```python
from build123d import *

# Parameters (mm, degrees)
SKETCH1_R           = 3
BOSS_EXTRUDE1_DEPTH = 10
BOSS_EXTRUDE2_START = -300
SKETCH2_R           = 3
BOSS_EXTRUDE2_DEPTH = 5
BOSS_EXTRUDE3_START = -270
SKETCH2_2_R         = 3
BOSS_EXTRUDE3_DEPTH = 5
SKETCH3_W           = 18
SKETCH3_H           = 5
BOSS_EXTRUDE5_DEPTH = 30
SKETCH4_R           = 3
CUT_EXTRUDE1_DEPTH  = 30


with BuildPart() as part:
    # Sketch1 → Boss-Extrude1 (new body)
    with BuildSketch(Plane(origin=(0, 0, 0), x_dir=(1, 0, 0), z_dir=(0, 1, 0))):
        with BuildLine():
            Line((-150, 100), (150, 100))
            Line((150, 100), (150, 0))
            ThreePointArc((150, 0), (0, -150), (-150, 0))
            Line((-150, 0), (-150, 100))
        make_face()
        Circle(SKETCH1_R, mode=Mode.SUBTRACT)
        with Locations((135, 0)):
            Circle(SKETCH1_R, mode=Mode.SUBTRACT)
        with Locations((134.486284242, -11.766025271)):
            Circle(SKETCH1_R, mode=Mode.SUBTRACT)
        with Locations((132.949046657, -23.442503985)):
            Circle(SKETCH1_R, mode=Mode.SUBTRACT)
        with Locations((130.399986549, -34.940571089)):
            Circle(SKETCH1_R, mode=Mode.SUBTRACT)
        with Locations((126.858503806, -46.172719349)):
            Circle(SKETCH1_R, mode=Mode.SUBTRACT)
        with Locations((122.35155125, -57.053465335)):
            Circle(SKETCH1_R, mode=Mode.SUBTRACT)
        with Locations((116.913429511, -67.5)):
            Circle(SKETCH1_R, mode=Mode.SUBTRACT)
        with Locations((110.585525979, -77.432818907)):
            Circle(SKETCH1_R, mode=Mode.SUBTRACT)
        with Locations((103.415999821, -86.776327308)):
            Circle(SKETCH1_R, mode=Mode.SUBTRACT)
        with Locations((95.45941546, -95.45941546)):
            Circle(SKETCH1_R, mode=Mode.SUBTRACT)
        with Locations((86.776327308, -103.415999821)):
            Circle(SKETCH1_R, mode=Mode.SUBTRACT)
        with Locations((77.432818907, -110.585525979)):
            Circle(SKETCH1_R, mode=Mode.SUBTRACT)
        with Locations((67.5, -116.913429511)):
            Circle(SKETCH1_R, mode=Mode.SUBTRACT)
        with Locations((57.053465335, -122.35155125)):
            Circle(SKETCH1_R, mode=Mode.SUBTRACT)
        with Locations((46.172719349, -126.858503806)):
            Circle(SKETCH1_R, mode=Mode.SUBTRACT)
        with Locations((34.940571089, -130.399986549)):
            Circle(SKETCH1_R, mode=Mode.SUBTRACT)
        with Locations((23.442503985, -132.949046657)):
            Circle(SKETCH1_R, mode=Mode.SUBTRACT)
        with Locations((11.766025271, -134.486284242)):
            Circle(SKETCH1_R, mode=Mode.SUBTRACT)
        with Locations((0, -135)):
            Circle(SKETCH1_R, mode=Mode.SUBTRACT)
        with Locations((-11.766025271, -134.486284242)):
            Circle(SKETCH1_R, mode=Mode.SUBTRACT)
        with Locations((-23.442503985, -132.949046657)):
            Circle(SKETCH1_R, mode=Mode.SUBTRACT)
        with Locations((-34.940571089, -130.399986549)):
            Circle(SKETCH1_R, mode=Mode.SUBTRACT)
        with Locations((-46.172719349, -126.858503806)):
            Circle(SKETCH1_R, mode=Mode.SUBTRACT)
        with Locations((-57.053465335, -122.35155125)):
            Circle(SKETCH1_R, mode=Mode.SUBTRACT)
        with Locations((-67.5, -116.913429511)):
            Circle(SKETCH1_R, mode=Mode.SUBTRACT)
        with Locations((-77.432818907, -110.585525979)):
            Circle(SKETCH1_R, mode=Mode.SUBTRACT)
        with Locations((-86.776327308, -103.415999821)):
            Circle(SKETCH1_R, mode=Mode.SUBTRACT)
        with Locations((-95.45941546, -95.45941546)):
            Circle(SKETCH1_R, mode=Mode.SUBTRACT)
        with Locations((-103.415999821, -86.776327308)):
            Circle(SKETCH1_R, mode=Mode.SUBTRACT)
        with Locations((-110.585525979, -77.432818907)):
            Circle(SKETCH1_R, mode=Mode.SUBTRACT)
        with Locations((-116.913429511, -67.5)):
            Circle(SKETCH1_R, mode=Mode.SUBTRACT)
        with Locations((-122.35155125, -57.053465335)):
            Circle(SKETCH1_R, mode=Mode.SUBTRACT)
        with Locations((-126.858503806, -46.172719349)):
            Circle(SKETCH1_R, mode=Mode.SUBTRACT)
        with Locations((-130.399986549, -34.940571089)):
            Circle(SKETCH1_R, mode=Mode.SUBTRACT)
        with Locations((-132.949046657, -23.442503985)):
            Circle(SKETCH1_R, mode=Mode.SUBTRACT)
        with Locations((-134.486284242, -11.766025271)):
            Circle(SKETCH1_R, mode=Mode.SUBTRACT)
        with Locations((-135, 0)):
            Circle(SKETCH1_R, mode=Mode.SUBTRACT)
    extrude(amount=BOSS_EXTRUDE1_DEPTH)

    # Sketch2 → Boss-Extrude2 (add)
    with BuildSketch(Plane.ZY.offset(150).offset(BOSS_EXTRUDE2_START)):
        Polygon((-25, 10), (-25, 35), (-30, 40), (-40, 40), (-45, 35), (-45, 10), align=None)
        with Locations((-35, 30)):
            Circle(SKETCH2_R, mode=Mode.SUBTRACT)
        with Locations((-35, 20)):
            Circle(SKETCH2_R, mode=Mode.SUBTRACT)
    extrude(amount=BOSS_EXTRUDE2_DEPTH)

    # Sketch2_2 → Boss-Extrude3 (add)
    with BuildSketch(Plane.ZY.offset(150).offset(BOSS_EXTRUDE3_START)):
        Polygon((-25, 10), (-25, 35), (-30, 40), (-40, 40), (-45, 35), (-45, 10), align=None)
        with Locations((-35, 30)):
            Circle(SKETCH2_2_R, mode=Mode.SUBTRACT)
        with Locations((-35, 20)):
            Circle(SKETCH2_2_R, mode=Mode.SUBTRACT)
    extrude(amount=-BOSS_EXTRUDE3_DEPTH)

    # Sketch3 → Boss-Extrude5 (add)
    with BuildSketch(Plane(origin=(0, 10, 0), x_dir=(1, 0, 0), z_dir=(0, 1, 0))):
        with Locations((135, 47.5)):
            Rectangle(SKETCH3_W, SKETCH3_H)
    extrude(amount=BOSS_EXTRUDE5_DEPTH)

    # Sketch4 → Cut-Extrude1 (cut)
    with BuildSketch(Plane.XY.offset(-45)):
        with Locations((135, 20)):
            Circle(SKETCH4_R)
        with Locations((135, 30)):
            Circle(SKETCH4_R)
        Polygon((126, 35), (131, 40), (126, 40), align=None)
        Polygon((139, 40), (144, 35), (144, 40), align=None)
    extrude(amount=-CUT_EXTRUDE1_DEPTH, mode=Mode.SUBTRACT)


solid = part.part
```
The model under review builds one solid part; all positions refer to its coordinate system, in mm. A direction names the side the tool comes from. Give positions to 0.01 mm unless a question says otherwise; leave off trailing zeros. Order: outer loops, then holes, each group sorted by start corner. A loop starts at its lowest first (then second) coordinate and runs counter-clockwise, first axis right, second up. Notation, with made-up numbers: (51, -3) - (105, -3) arc R33 ccw to (105, 32) - close; hole circle Ø1 at (-38, 45.5). An arc over 180 degrees is marked (long way). Use CSV: the item, a comma, the result in double quotes. Start each with the question number.
Q1. The part is to be moulded in two halves that separate along Z. For faces 3 (the flat face through (145, 25, -35)), 4 (the cylindrical face through (3.298, 4.93, 149.964)), 5 (the cylindrical face through (-129.016, 4.93, 37.602)), say which applies: +Z half, -Z half, draft (parallel to the pull), parting line (faces both ways), or undercut.
Q2. Tool access review of faces 1 (the flat face through (120, 25, -35)), 2 (the cylindrical face through (-125.47, 4.93, 48.83)): name each direction out of +Z, -Z, +X, -X, +Y, -Y from which nothing blocks a thin tool from reaching the whole face with its end or side.
Q3. To check wall thickness, follow line 1 along X through (y, z) = (7, 9); line 2 along Y through (x, z) = (45, -32.5); line 3 along Z through (x, y) = (-47, 6). State the ranges of each line that lie inside material, in increasing order. Write a range as [from, to].
Q4. We need section A-A, the plane z = -8.5. Write out the cut boundary in (x, y), and give its area (3 significant figures).
Q5. Clearance check with flat-ended pins moving along their axes: pin 1 Ø9.5 at (x, z) = (-67.5, 116.91) entering from +Y; pin 2 Ø3.5 at (x, z) = (67.5, 116.91) entering from -Y; pin 3 Ø20 at (x, y) = (136, 27.5) entering from -Z; pin 4 Ø10 at (y, z) = (28, -33) entering from -X. State where each tip first meets the part, or that it passes through.
Outcome:
1,face 3,"draft"
1,face 4,"+Z half"
1,face 5,"undercut"
2,face 1,"+Z, -Z, -X, +Y"
2,face 2,"+Y, -Y"
3,line 1,"x = [-149.73, -135.65], [-133.32, 133.32], [135.65, 149.73]"
3,line 2,"y = [0, 10]"
3,line 3,"z = [-100, 123.97], [129.74, 142.45]"
4,outline,"(-150, 0) - (150, 0) - (150, 10) - (-150, 10) - close"
4,area,"3,000 mm^2"
5,pin 1,"stops at y = 10"
5,pin 2,"passes through"
5,pin 3,"stops at z = -50"
5,pin 4,"stops at x = 120"
